Source: three-view drawing plus pictorial views. Frame: mm from the lowest corner of the part. Round coordinates to 2 decimals unless told otherwise and drop trailing zeros. Loops run counter-clockwise (first coordinate to the right, second up) from the corner with the lowest first, then second, coordinate; pieces in that order, holes last. Notation, with made-up numbers: M 50.25,5.5 L 105.25,5.5 A24 cw 105.25,31.5 Z; hole C 45,49 d6. An arc over 180 degrees is marked long. Return JSON: item names as keys, results as strings. Group by question number.
1) Section B-B (z = 19.05). Output: boundary loops of the cut face in (x, y) (3 decimals).
2) Section A-A (x = 2.54). Output: boundary loops of the cut face in (y, z) (3 decimals).
3) Section D-D (z = 34). Output: boundary loops of the cut face in (x, y) (3 decimals), plus the area to 3 significant figures.
4) Section C-C (y = 2.1). Output: boundary loops of the cut face in (x, z) (3 decimals), plus the area to 3 significant figures.
5) Material intervals for line 1 (X direction, y = 1.4, z = 19.05); line 2 (Z direction, x = 20.5, y = 2.55) (3 decimals); line 3 (X direction, y = 1, z = 10.5), sorted ascending. Write a range as from..to.
6) Contact query for a flat-ended pin moving along its axis: P1, Ø1, axis at y = 1.5, z = 7, coming from the +X side. Output: stop coordinate, or through.
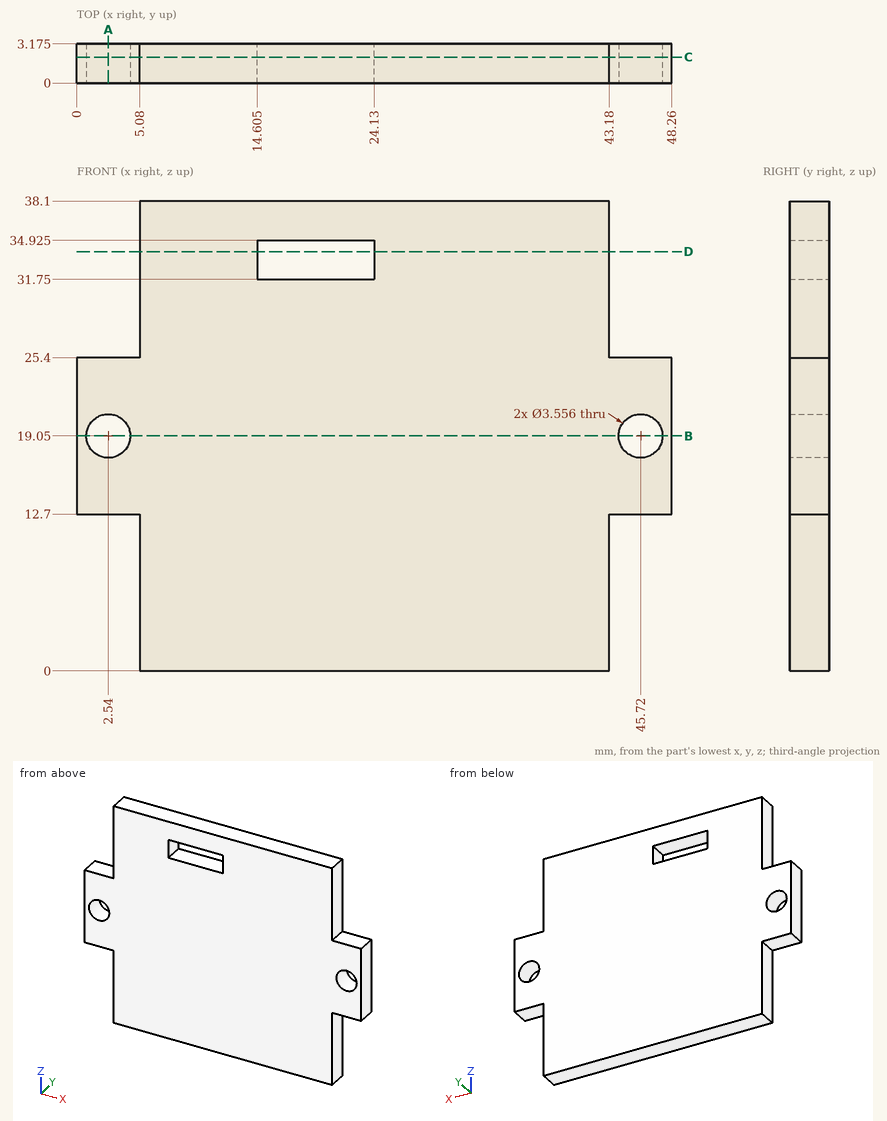
Returned:
{
 "1": {"outline": "M 0,0 L 0.762,0 L 0.762,3.175 L 0,3.175 Z; M 4.318,0 L 43.942,0 L 43.942,3.175 L 4.318,3.175 Z; M 47.498,0 L 48.26,0 L 48.26,3.175 L 47.498,3.175 Z"},
 "2": {"outline": "M 0,12.7 L 3.175,12.7 L 3.175,17.272 L 0,17.272 Z; M 0,20.828 L 3.175,20.828 L 3.175,25.4 L 0,25.4 Z"},
 "3": {"outline": "M 5.08,0 L 14.605,0 L 14.605,3.175 L 5.08,3.175 Z; M 24.13,0 L 43.18,0 L 43.18,3.175 L 24.13,3.175 Z", "area": "90.7 mm^2"},
 "4": {"outline": "M 0,12.7 L 5.08,12.7 L 5.08,0 L 43.18,0 L 43.18,12.7 L 48.26,12.7 L 48.26,25.4 L 43.18,25.4 L 43.18,38.1 L 5.08,38.1 L 5.08,25.4 L 0,25.4 Z; hole C 2.54,19.05 d3.556; hole M 14.605,31.75 L 24.13,31.75 L 24.13,34.925 L 14.605,34.925 Z; hole C 45.72,19.05 d3.556", "area": "1,530 mm^2"},
 "5": {"line 1": "x = 0..0.76, 4.32..43.94, 47.5..48.26", "line 2": "z = 0..31.75, 34.925..38.1", "line 3": "x = 5.08..43.18"},
 "6": {"P1": "stops at x = 43.18"}
}
